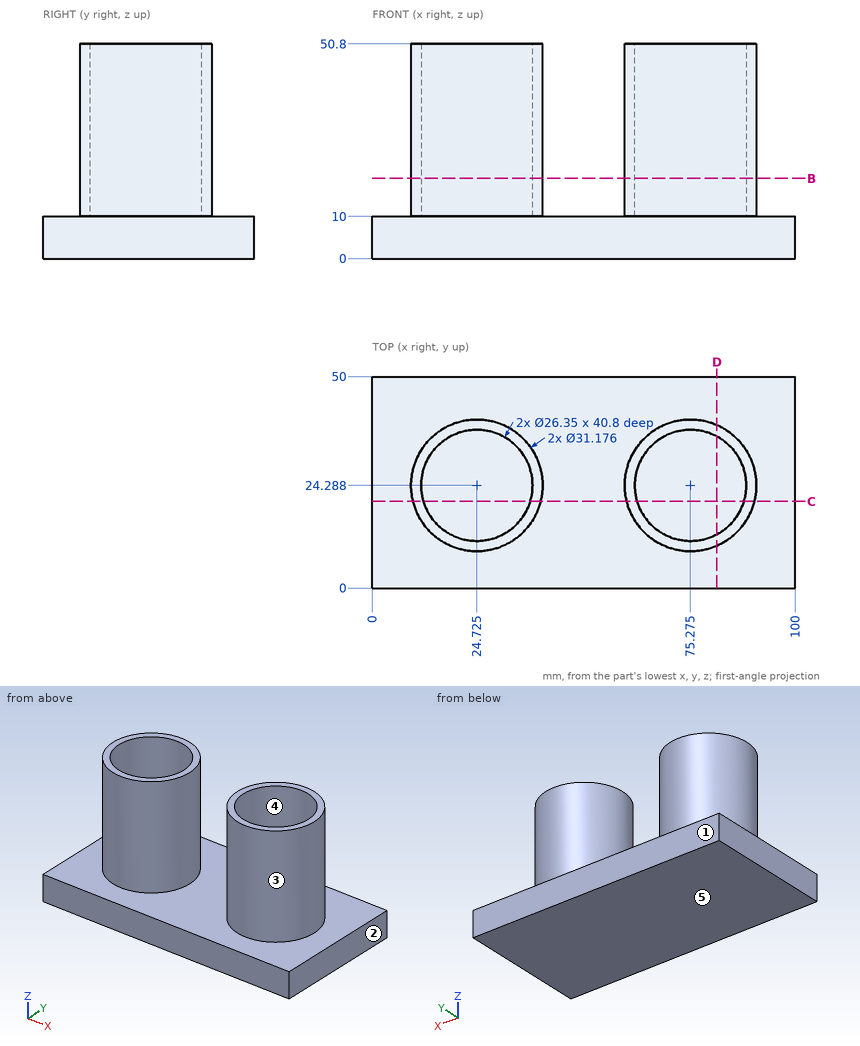
Check sheet for the drawn part. Datum: minimum x, y, z corner. Units: mm. A direction names the side the tool comes from. Round coordinates to 2 decimals unless told otherwise and drop trailing zeros. Loops run counter-clockwise (first coordinate to the right, second up) from the corner with the lowest first, then second, coordinate; pieces in that order, holes last. Notation, with made-up numbers: (36.5, -36) - (45.5, -36) arc R17 ccw to (45.5, -24) - close; hole circle Ø9 at (-40, 63.5). An arc over 180 degrees is marked (long way). Use one line per item in the form item = value.
1. Section check B-B on z = 19. Give the number of separate pieces and of enclosed holes in the cut face, and give its area (3 significant figures).
A:
separate_pieces = 2
enclosed_holes = 2
area = 436 mm²
2. Section check D-D on x = 81.5. Record the cut outline in (y, z).
A:
outline = (0, 0) - (50, 0) - (50, 10) - (38.58, 10) - (38.58, 50.8) - (35.9, 50.8) - (35.9, 10) - (12.68, 10) - (12.68, 50.8) - (10, 50.8) - (10, 10) - (0, 10) - close
3. Section check C-C on y = 20.5. Record the cut outline in (x, z) (1 decimal).
A:
outline = (0, 0) - (100, 0) - (100, 10) - (90.4, 10) - (90.4, 50.8) - (87.9, 50.8) - (87.9, 10) - (62.7, 10) - (62.7, 50.8) - (60.2, 50.8) - (60.2, 10) - (39.8, 10) - (39.8, 50.8) - (37.3, 50.8) - (37.3, 10) - (12.1, 10) - (12.1, 50.8) - (9.6, 50.8) - (9.6, 10) - (0, 10) - close
4. Access from +Z, -Z, +X, -X, +Y, -Y to the whole of each face (thin tool, end or side, straight path). Record for the marked faces 4 and 5.
A:
face_4 = +Z
face_5 = -Z, +X, -X, +Y, -Y
5. Gauge pin test, flat ends, axial feed: pin 1 Ø21 at (x, y) = (22, 28.5) entering from +Z; pin 2 Ø4 at (x, z) = (72.5, 40) entering from -Y; pin 3 Ø1.5 at (x, y) = (49, 20) entering from +Z; pin 4 Ø6 at (y, z) = (23, 42) entering from +X. Record the tip position at first contact, or that the pin passes through.
A:
pin_1 = 50.8
pin_2 = 8.72
pin_3 = 10
pin_4 = 90.86
6. Scan lines: probe 1 along X at (y, z) = (23, 25.5); probe 2 along X at (y, z) = (14.5, 28) (1 decimal); probe 3 along Z at (x, y) = (20, 9). Record each from-to range of solid material in increasing order.
A:
probe_1 = 9.19 to 11.61, 37.84 to 40.26, 59.74 to 62.16, 88.39 to 90.81
probe_2 = 12.6 to 15.9, 33.5 to 36.9, 63.1 to 66.5, 84.1 to 87.4
probe_3 = 0 to 10
7. Draft check along X on the marked faces 1, 2 and 3. Enter one of: pulls with the +X half, pulls with the -X half, needs draft (parallel to the pull), parting line crosses it, or undercut.
A:
face_1 = needs draft
face_2 = pulls with the +X half
face_3 = undercut
